Model file for the job. Use its own axes, mm. Coordinates: 2 decimals unless noted, no trailing zeros. Order: outer loops, then holes, each group sorted by start corner. A loop starts at its lowest first (then second) coordinate and runs counter-clockwise, first axis right, second up.
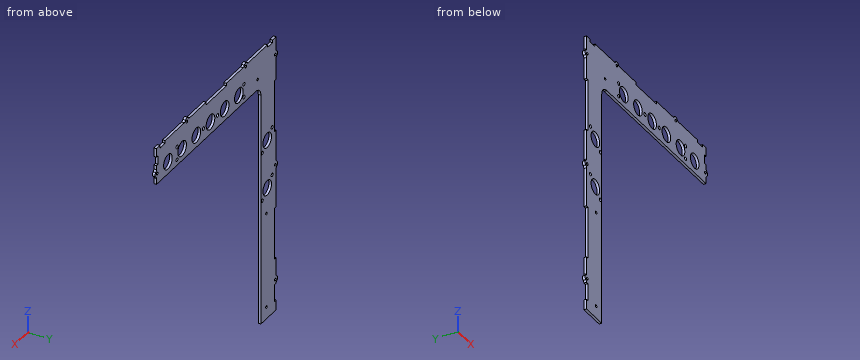
from build123d import *

# Parameters (mm, degrees)
EXTRUDE_1_DEPTH        = 3
SKETCH_2_W             = 3
SKETCH_2_H             = 10
CUT_EXTRUDE_1_DEPTH    = 3
SKETCH_4_W             = 3
SKETCH_4_H             = 3
FILLET_1_R             = 3
SKETCH_5_R             = 1.5
CUT_EXTRUDE_2_DEPTH    = 3
SKETCH_6_W             = 10
SKETCH_6_H             = 3
CUT_EXTRUDE_3_DEPTH    = 3
SKETCH_7_W             = 40
SKETCH_7_H             = 3
CUT_EXTRUDE_4_DEPTH    = 3
SKETCH_9_W             = 3
SKETCH_9_H             = 60
SKETCH_9_H_2           = 20
CUT_EXTRUDE_5_DEPTH    = 3
SKETCH_11_W            = 3
SKETCH_11_H            = 3
SKETCH_12_W            = 3
SKETCH_12_H            = 3
SKETCH_13_R            = 1.5
CUT_EXTRUDE_6_DEPTH    = 3
FILLET_2_R             = 3
SKETCH_14_W            = 3
SKETCH_14_H            = 3
SKETCH_15_W            = 3
SKETCH_15_H            = 3
SKETCH_16_W            = 3
SKETCH_16_H            = 3
FILLET_3_R             = 3
SKETCH_17_R            = 1.5
CUT_EXTRUDE_7_DEPTH    = 3
SKETCH_18_R            = 8.5
CUT_EXTRUDE_8_DEPTH    = 3
PATTERN_LINEAR_2_COUNT = 6
PATTERN_LINEAR_2_PITCH = 28
SKETCH_19_R            = 8.5
CUT_EXTRUDE_9_DEPTH    = 3
SKETCH_20_R            = 8.5
CUT_EXTRUDE_10_DEPTH   = 3
FILLET_4_R             = 10
SKETCH_21_R            = 2
CUT_EXTRUDE_11_DEPTH   = 3
SKETCH_22_R            = 1.9
CUT_EXTRUDE_12_DEPTH   = 3
SKETCH_23_R            = 1.5
CUT_EXTRUDE_13_DEPTH   = 3
SKETCH_24_R            = 1.5
CUT_EXTRUDE_14_DEPTH   = 3


with BuildPart() as part:
    # Эскиз1 → Бобышка-Вытянуть1 (new body)
    with BuildSketch(Plane(origin=(0, 0, 0), x_dir=(1, 0, 0), z_dir=(0, 1, 0))):
        Polygon((0, 0), (0, 321.5), (30, 321.5), (30, 42), (236, 42), (236, 0), align=None)
    extrude(amount=EXTRUDE_1_DEPTH)

    # Эскиз2 → Вырез-Вытянуть1 (cut)
    with BuildSketch(Plane(origin=(0, 3, 0), x_dir=(1, 0, 0), z_dir=(0, 1, 0))):
        with Locations((234.5, 15)):
            Rectangle(SKETCH_2_W, SKETCH_2_H)
    extrude(amount=-CUT_EXTRUDE_1_DEPTH, mode=Mode.SUBTRACT)

    # Эскиз4 → Повернуть1 (revolve)
    with BuildSketch(Plane(origin=(236, 0, 0), x_dir=(0, 0, -1), z_dir=(1, 0, 0))):
        with Locations((31.5, 1.5)):
            Rectangle(SKETCH_4_W, SKETCH_4_H)
    revolve(axis=Axis((236, 0, -30), (0, 1, 0)))

    # Скругление1
    fillet_1_edges = [part.edges().sort_by_distance(p)[0] for p in [
        (236, 1.5, -33),
        (236, 1.5, -27),
    ]]
    fillet(fillet_1_edges, radius=FILLET_1_R)

    # Эскиз5 → Вырез-Вытянуть2 (cut)
    with BuildSketch(Plane(origin=(0, 3, 0), x_dir=(1, 0, 0), z_dir=(0, 1, 0))):
        with Locations(Location((234.5, 30, 0), (0, 0, 270))):
            Circle(SKETCH_5_R)
    extrude(amount=-CUT_EXTRUDE_2_DEPTH, mode=Mode.SUBTRACT)

    # Эскиз6 → Вырез-Вытянуть3 (cut)
    with BuildSketch(Plane(origin=(0, 3, 0), x_dir=(1, 0, 0), z_dir=(0, 1, 0))):
        with Locations((224, 1.5)):
            Rectangle(SKETCH_6_W, SKETCH_6_H)
        with Locations((12, 1.5)):
            Rectangle(SKETCH_6_W, SKETCH_6_H)
    extrude(amount=-CUT_EXTRUDE_3_DEPTH, mode=Mode.SUBTRACT)

    # Эскиз7 → Вырез-Вытянуть4 (cut)
    with BuildSketch(Plane(origin=(0, 3, 0), x_dir=(1, 0, 0), z_dir=(0, 1, 0))):
        with Locations((118, 1.5)):
            Rectangle(SKETCH_7_W, SKETCH_7_H)
    extrude(amount=-CUT_EXTRUDE_4_DEPTH, mode=Mode.SUBTRACT)

    # Эскиз9 → Вырез-Вытянуть5 (cut)
    with BuildSketch(Plane(origin=(0, 3, 0), x_dir=(1, 0, 0), z_dir=(0, 1, 0))):
        with Locations((1.5, 80)):
            Rectangle(SKETCH_9_W, SKETCH_9_H)
        with Locations((1.5, 230)):
            Rectangle(SKETCH_9_W, SKETCH_9_H)
        with Locations((1.5, 300)):
            Rectangle(SKETCH_9_W, SKETCH_9_H_2)
    extrude(amount=-CUT_EXTRUDE_5_DEPTH, mode=Mode.SUBTRACT)

    # Эскиз11 → Повернуть2 (revolve)
    with BuildSketch(Plane.XY):
        with Locations((61.5, 1.5)):
            Rectangle(SKETCH_11_W, SKETCH_11_H)
    revolve(axis=Axis((60, 0, 0), (0, 1, 0)))

    # Эскиз12 → Повернуть3 (revolve)
    with BuildSketch(Plane.XY):
        with Locations((174.5, 1.5)):
            Rectangle(SKETCH_12_W, SKETCH_12_H)
    revolve(axis=Axis((176, 0, 0), (0, 1, 0)))

    # Эскиз13 → Вырез-Вытянуть6 (cut)
    with BuildSketch(Plane(origin=(0, 3, 0), x_dir=(1, 0, 0), z_dir=(0, 1, 0))):
        with Locations(Location((60, 1.5, 0), (0, 0, 270))):
            Circle(SKETCH_13_R)
        with Locations(Location((176, 1.5, 0), (0, 0, 270))):
            Circle(SKETCH_13_R)
    extrude(amount=-CUT_EXTRUDE_6_DEPTH, mode=Mode.SUBTRACT)

    # Скругление2
    fillet_2_edges = [part.edges().sort_by_distance(p)[0] for p in [
        (63, 1.5, 0),
        (57, 1.5, 0),
        (179, 1.5, 0),
        (173, 1.5, 0),
    ]]
    fillet(fillet_2_edges, radius=FILLET_2_R)

    # Эскиз14 → Повернуть4 (revolve)
    with BuildSketch(Plane.ZY):
        with Locations((-286.5, 1.5)):
            Rectangle(SKETCH_14_W, SKETCH_14_H)
    revolve(axis=Axis((0, 0, -285), (0, 1, 0)))

    # Эскиз15 → Повернуть5 (revolve)
    with BuildSketch(Plane.ZY):
        with Locations((-151.5, 1.5)):
            Rectangle(SKETCH_15_W, SKETCH_15_H)
    revolve(axis=Axis((0, 0, -150), (0, 1, 0)))

    # Эскиз16 → Повернуть6 (revolve)
    with BuildSketch(Plane.ZY):
        with Locations((-21.5, 1.5)):
            Rectangle(SKETCH_16_W, SKETCH_16_H)
    revolve(axis=Axis((0, 0, -20), (0, 1, 0)))

    # Скругление3
    # the kernel refuses this fillet: 3 mm, written as the material it adds along each edge
    with BuildSketch(Plane(origin=(0, 3, -282), x_dir=(-0.9659258262890682, 0, -0.2588190451025208), z_dir=(0, -1, 0)), Plane(origin=(0, 3, -147), x_dir=(-0.9659258262890682, 0, -0.2588190451025208), z_dir=(0, -1, 0))) as fillet_3_piece_1:
        with BuildLine():
            CenterArc((2.329371406, -2.897777479), FILLET_3_R, 105, 60)
            Line((-0.568406073, -2.121320344), (-0.626361623, -2.105791201))
            Line((-0.626361623, -2.105791201), (-0.05795555, 0.015529143))
            Line((-0.05795555, 0.015529143), (0.015529143, 0.05795555))
            ThreePointArc((0.015529143, 0.05795555), (0.776457135, -0.042222521), (1.537385128, 0.05795555))
            Line((1.537385128, 0.05795555), (1.552914271, 0))
        make_face()
    extrude(amount=3)
    with BuildSketch(Plane(origin=(0, 3, -288), x_dir=(0, 0, -1), z_dir=(0, -1, 0))) as fillet_3_piece_2:
        with BuildLine():
            CenterArc((2.2, -2.993325909), FILLET_3_R, 93.822553729, 56.251011404)
            Line((-0.4, -1.496662955), (-0.452, -1.466729696))
            ThreePointArc((-0.452, -1.466729696), (-0.159690158, -0.759104736), (-0.06, 0))
            Line((-0.06, 0), (0, 0.06))
            ThreePointArc((0, 0.06), (1, 0.06), (1.996, 0.059866518))
            Line((1.996, 0.059866518), (2, 0))
        make_face()
    extrude(amount=3)
    with BuildSketch(Plane(origin=(0, 3, -153), x_dir=(0, 0, -1), z_dir=(0, -1, 0)), Plane(origin=(0, 3, -23), x_dir=(0, 0, -1), z_dir=(0, -1, 0))) as fillet_3_piece_3:
        with BuildLine():
            CenterArc((2.196152423, -3), FILLET_3_R, 90, 60)
            Line((-0.401923789, -1.5), (-0.453885313, -1.47))
            ThreePointArc((-0.453885313, -1.47), (-0.160178071, -0.760927993), (-0.06, 0))
            Line((-0.06, 0), (0, 0.06))
            Line((0, 0.06), (2.196152423, 0.06))
            Line((2.196152423, 0.06), (2.196152423, 0))
        make_face()
    extrude(amount=3)
    with BuildSketch(Plane(origin=(0, 3, -17), x_dir=(0, 0, 1), z_dir=(0, -1, 0))) as fillet_3_piece_4:
        with BuildLine():
            CenterArc((2.196152423, 3), FILLET_3_R, 210, 60)
            Line((-0.401923789, 1.5), (-0.453885313, 1.47))
            ThreePointArc((-0.453885313, 1.47), (-0.160178071, 0.760927993), (-0.06, 0))
            Line((-0.06, 0), (0, -0.06))
            Line((0, -0.06), (2.196152423, -0.06))
            Line((2.196152423, -0.06), (2.196152423, 0))
        make_face()
    extrude(amount=3)

    # Эскиз17 → Вырез-Вытянуть7 (cut)
    with BuildSketch(Plane(origin=(0, 3, 0), x_dir=(1, 0, 0), z_dir=(0, 1, 0))):
        with Locations(Location((1.5, 20, 0), (0, 0, 270))):
            Circle(SKETCH_17_R)
        with Locations(Location((1.5, 150, 0), (0, 0, 270))):
            Circle(SKETCH_17_R)
        with Locations(Location((1.5, 285, 0), (0, 0, 270))):
            Circle(SKETCH_17_R)
    extrude(amount=-CUT_EXTRUDE_7_DEPTH, mode=Mode.SUBTRACT)

    # Эскиз18 → Вырез-Вытянуть8 (cut)
    with BuildSketch(Plane(origin=(0, 3, 0), x_dir=(1, 0, 0), z_dir=(0, 1, 0))):
        with Locations(Location((213.5, 28, 0), (0, 0, 270))):
            Circle(SKETCH_18_R)
    cut_extrude_8 = extrude(amount=-CUT_EXTRUDE_8_DEPTH, mode=Mode.SUBTRACT)

    # Линейный массив2: Вырез-Вытянуть8 ×6
    with Locations(*[(-i * PATTERN_LINEAR_2_PITCH, 0, 0) for i in range(1, PATTERN_LINEAR_2_COUNT)]):
        add(cut_extrude_8, mode=Mode.SUBTRACT)

    # Эскиз19 → Вырез-Вытянуть9 (cut)
    with BuildSketch(Plane(origin=(0, 3, 0), x_dir=(1, 0, 0), z_dir=(0, 1, 0))):
        with Locations(Location((17.5, 112, 0), (0, 0, 270))):
            Circle(SKETCH_19_R)
    extrude(amount=-CUT_EXTRUDE_9_DEPTH, mode=Mode.SUBTRACT)

    # Эскиз20 → Вырез-Вытянуть10 (cut)
    with BuildSketch(Plane(origin=(0, 3, 0), x_dir=(1, 0, 0), z_dir=(0, 1, 0))):
        with Locations(Location((17.5, 168, 0), (0, 0, 270))):
            Circle(SKETCH_20_R)
    extrude(amount=-CUT_EXTRUDE_10_DEPTH, mode=Mode.SUBTRACT)

    # Скругление4
    fillet_4_edges = [part.edges().sort_by_distance(p)[0] for p in [
        (30, 1.5, -42),
    ]]
    fillet(fillet_4_edges, radius=FILLET_4_R)

    # Эскиз21 → Вырез-Вытянуть11 (cut)
    with BuildSketch(Plane(origin=(0, 3, 0), x_dir=(1, 0, 0), z_dir=(0, 1, 0))):
        with Locations(Location((115.5, 28, 0), (0, 0, 270))):
            Circle(SKETCH_21_R)
        with Locations(Location((143.5, 28, 0), (0, 0, 270))):
            Circle(SKETCH_21_R)
        with Locations(Location((195.5, 35.5, 0), (0, 0, 270))):
            Circle(SKETCH_21_R)
        with Locations(Location((195.5, 20.5, 0), (0, 0, 270))):
            Circle(SKETCH_21_R)
        with Locations(Location((63.5, 35.5, 0), (0, 0, 270))):
            Circle(SKETCH_21_R)
        with Locations(Location((63.5, 20.5, 0), (0, 0, 270))):
            Circle(SKETCH_21_R)
    extrude(amount=-CUT_EXTRUDE_11_DEPTH, mode=Mode.SUBTRACT)

    # Эскиз22 → Вырез-Вытянуть12 (cut)
    with BuildSketch(Plane(origin=(0, 3, 0), x_dir=(1, 0, 0), z_dir=(0, 1, 0))):
        with Locations(Location((27.222718241, 121.722718241, 0), (0, 0, 270))):
            Circle(SKETCH_22_R)
        with Locations(Location((7.777281759, 102.277281759, 0), (0, 0, 270))):
            Circle(SKETCH_22_R)
        with Locations(Location((27.222718241, 177.722718241, 0), (0, 0, 270))):
            Circle(SKETCH_22_R)
        with Locations(Location((7.777281759, 158.277281759, 0), (0, 0, 270))):
            Circle(SKETCH_22_R)
    extrude(amount=-CUT_EXTRUDE_12_DEPTH, mode=Mode.SUBTRACT)

    # Эскиз23 → Вырез-Вытянуть13 (cut)
    with BuildSketch(Plane(origin=(0, 3, 0), x_dir=(1, 0, 0), z_dir=(0, 1, 0))):
        with Locations(Location((19, 307.5, 0), (0, 0, 270))):
            Circle(SKETCH_23_R)
        with Locations(Location((19, 197.5, 0), (0, 0, 270))):
            Circle(SKETCH_23_R)
    extrude(amount=-CUT_EXTRUDE_13_DEPTH, mode=Mode.SUBTRACT)

    # Эскиз24 → Вырез-Вытянуть14 (cut)
    with BuildSketch(Plane(origin=(0, 3, 0), x_dir=(1, 0, 0), z_dir=(0, 1, 0))):
        with Locations(Location((36.5, 30, 0), (0, 0, 270))):
            Circle(SKETCH_24_R)
    extrude(amount=-CUT_EXTRUDE_14_DEPTH, mode=Mode.SUBTRACT)


solid = part.part
Q1. Cut at B-B, the plane x = 213.5. List the corners of the cut face in (y, z).
Established:
outline: (0, -42) - (3, -42) - (3, -36.5) - (0, -36.5) - close; (0, -19.5) - (3, -19.5) - (3, 0) - (0, 0) - close
Q2. Cut at C-C, the plane z = -238.5. List the corners of the cut face in (x, y), plus the area to 3 significant figures.
Established:
outline: (3, 0) - (30, 0) - (30, 3) - (3, 3) - close
area: 81.0 mm2
Q3. Cut at A-A, the plane x = 101.5. List the corners of the cut face in (y, z), plus the area to 3 significant figures.
Established:
outline: (0, -42) - (3, -42) - (3, -36.5) - (0, -36.5) - close; (0, -19.5) - (3, -19.5) - (3, -3) - (0, -3) - close
area: 66.0 mm2
Q4. Probe line 1 (Z direction, x = 95, y = 0.85); line 2 (Z direction, x = 176, y = 1.75); line 3 (X direction, y = 2, z = -112). List the from-to ranges inside material, lowest first.
Established:
line 1: z = -42 to -33.48, -22.52 to 0
line 2: z = -42 to -3, 0 to 3
line 3: x = 0 to 9, 26 to 30
Q5. Drop flat-ended pins along their axis: P1, Ø0.9, axis at y = 1.5, z = -16.5, coming from the +X side; P2, Ø1, axis at y = 2.5, z = -164.5, coming from the -X side; P3, Ø1.5, axis at y = 2, z = -43.5, coming from the +X side; P4, Ø15.5, axis at x = 73.5, z = -28, coming from the -Y side. Give the stop position or say it passes through.
Established:
P1: stops at x = 233
P2: stops at x = 0
P3: stops at x = 36.2
P4: passes through
Q6. Cut at D-D, the plane y = 2.2. Count the separate pieces of the cut face and the enclosed holes in it, plus the area to 3 significant figures.
Established:
separate pieces: 1
enclosed holes: 27
area: 15,800 mm2
